from build123d import *

# Parameters (mm, degrees)
SKETCH1_R           = 1.5
SKETCH1_W           = 15.5
SKETCH1_H           = 15.5
BOSS_EXTRUDE1_DEPTH = 1.6
CUT_EXTRUDE2_DEPTH  = 91.713045172
FILLET2_R           = 3
FILLET3_R           = 3


with BuildPart() as part:
    # Sketch1 → Boss-Extrude1 (new body)
    with BuildSketch(Plane.XY):
        with BuildLine():
            Line((80.807032999, -9.202000204), (80.807032999, 37.709242496))
            ThreePointArc((80.807032999, 37.709242496), (79.927673142, 39.831242844), (77.805109389, 40.709241907))
            Line((77.805109389, 40.709241907), (-72.154484411, 40.613083107))
            ThreePointArc((-72.154484411, 40.613083107), (-74.271159988, 39.737121752), (-75.152545414, 37.622699011))
            Line((-75.152545414, 37.622699011), (-75.383320814, -34.379217889))
            ThreePointArc((-75.383320814, -34.379217889), (-74.508053368, -36.506751286), (-72.383336219, -37.388833194))
            Line((-72.383336219, -37.388833194), (-25.613726719, -37.388833194))
            ThreePointArc((-25.613726719, -37.388833194), (-25.488077715, -37.391465627), (-25.362649219, -37.399358309))
            Line((-25.362649219, -37.399358309), (19.631715181, -41.178308109))
            ThreePointArc((19.631715181, -41.178308109), (19.757143676, -41.18620079), (19.88279268, -41.188833223))
            Line((19.88279268, -41.188833223), (68.14475528, -41.188833223))
            ThreePointArc((68.14475528, -41.188833223), (69.898886106, -40.622559803), (70.990805162, -39.137516598))
            Line((70.990805162, -39.137516598), (80.653082862, -10.150683598))
            ThreePointArc((80.653082862, -10.150683598), (80.768295364, -9.682546983), (80.807032999, -9.202000204))
        make_face()
        with Locations((-19.612967014, -21.188833189)):
            Circle(SKETCH1_R, mode=Mode.SUBTRACT)
        with Locations((7.057032986, -25.938833189)):
            Circle(SKETCH1_R, mode=Mode.SUBTRACT)
        with Locations((43.657032986, 35.811166811)):
            Circle(SKETCH1_R, mode=Mode.SUBTRACT)
        with Locations((-70.817967014, -7.888833189)):
            Circle(SKETCH1_R, mode=Mode.SUBTRACT)
        with Locations((57.907032986, -7.888833189)):
            Circle(SKETCH1_R, mode=Mode.SUBTRACT)
        with Locations((-51.342967014, 18.711166811)):
            Circle(SKETCH1_R, mode=Mode.SUBTRACT)
        with Locations((-64.642967014, 30.111166811)):
            Rectangle(SKETCH1_W, SKETCH1_H, mode=Mode.SUBTRACT)
        with Locations((-45.642967014, 30.111166811)):
            Rectangle(SKETCH1_W, SKETCH1_H, mode=Mode.SUBTRACT)
        with Locations((-26.642967014, 30.111166811)):
            Rectangle(SKETCH1_W, SKETCH1_H, mode=Mode.SUBTRACT)
        with Locations((-7.642967014, 30.111166811)):
            Rectangle(SKETCH1_W, SKETCH1_H, mode=Mode.SUBTRACT)
        with Locations((11.357032986, 30.111166811)):
            Rectangle(SKETCH1_W, SKETCH1_H, mode=Mode.SUBTRACT)
        with Locations((30.357032986, 30.111166811)):
            Rectangle(SKETCH1_W, SKETCH1_H, mode=Mode.SUBTRACT)
        with Locations((-62.267967014, 11.111166811)):
            Rectangle(SKETCH1_W, SKETCH1_H, mode=Mode.SUBTRACT)
        with Locations((-40.892967014, 11.111166811)):
            Rectangle(SKETCH1_W, SKETCH1_H, mode=Mode.SUBTRACT)
        with Locations((-21.892967014, 11.111166811)):
            Rectangle(SKETCH1_W, SKETCH1_H, mode=Mode.SUBTRACT)
        with Locations((-2.892967014, 11.111166811)):
            Rectangle(SKETCH1_W, SKETCH1_H, mode=Mode.SUBTRACT)
        with Locations((16.107032986, 11.111166811)):
            Rectangle(SKETCH1_W, SKETCH1_H, mode=Mode.SUBTRACT)
        with Locations((35.107032986, 11.111166811)):
            Rectangle(SKETCH1_W, SKETCH1_H, mode=Mode.SUBTRACT)
        with Locations((-57.517967014, -7.888833189)):
            Rectangle(SKETCH1_W, SKETCH1_H, mode=Mode.SUBTRACT)
        with Locations((-31.392967014, -7.888833189)):
            Rectangle(SKETCH1_W, SKETCH1_H, mode=Mode.SUBTRACT)
        with Locations((-12.392967014, -7.888833189)):
            Rectangle(SKETCH1_W, SKETCH1_H, mode=Mode.SUBTRACT)
        with Locations((6.607032986, -7.888833189)):
            Rectangle(SKETCH1_W, SKETCH1_H, mode=Mode.SUBTRACT)
        with Locations((25.607032986, -7.888833189)):
            Rectangle(SKETCH1_W, SKETCH1_H, mode=Mode.SUBTRACT)
        with Locations((44.607032986, -7.888833189)):
            Rectangle(SKETCH1_W, SKETCH1_H, mode=Mode.SUBTRACT)
        with Locations((-62.267967014, -26.888833189)):
            Rectangle(SKETCH1_W, SKETCH1_H, mode=Mode.SUBTRACT)
        with Locations((-38.612967014, -26.888833189)):
            Rectangle(SKETCH1_W, SKETCH1_H, mode=Mode.SUBTRACT)
        with Locations((26.057032986, -30.688833189)):
            Rectangle(SKETCH1_W, SKETCH1_H, mode=Mode.SUBTRACT)
        with Locations((55.057032986, -30.688833189)):
            Rectangle(SKETCH1_W, SKETCH1_H, mode=Mode.SUBTRACT)
    extrude(amount=BOSS_EXTRUDE1_DEPTH)

    # Sketch3 → Cut-Extrude2 (cut, through all)
    with BuildSketch(Plane.XY.offset(1.6)):
        Polygon((47.443249451, 42.560753869), (47.443249451, 3.300099698), (61.120116682, 3.300099698), (61.120116682, -19.548313794), (65.786341973, -19.548313794), (65.786341973, -41.188833223), (73.358886795, -43.51481274), (105.294000543, 60.45432308), align=None)
    extrude(amount=-CUT_EXTRUDE2_DEPTH, mode=Mode.SUBTRACT)

    # Fillet2
    fillet2_edges = [part.edges().sort_by_distance(p)[0] for p in [
        (47.443249451, 40.689772929, 0.8),
        (65.786341973, -19.548313794, 0.8),
        (61.120116682, 3.300099698, 0.8),
    ]]
    fillet(fillet2_edges, radius=FILLET2_R)

    # Fillet3
    fillet3_edges = [part.edges().sort_by_distance(p)[0] for p in [
        (65.786341973, -41.188833223, 0.8),
    ]]
    fillet(fillet3_edges, radius=FILLET3_R)


solid = part.part
Read the model definition and answer for the solid it produces. Units are mm, in the model's axes. Round coordinates to 2 decimals unless told otherwise and drop trailing zeros. Order: outer loops, then holes, each group sorted by start corner. A loop starts at its lowest first (then second) coordinate and runs counter-clockwise, first axis right, second up.
1) Straight lines are drawn through the part: L1, parallel to Y at x = -59, z = 1.4; L2, parallel to Y at x = -27.5, z = 1.35; L3, parallel to X at y = -31.5, z = 0.6. For each, find the intervals that lie inside material, in ascending order.
2) The mould has two halves that part along X. Classify faces 1 (the face through (-74.25, 39.76, 0.79)), 2 (the face through (-52.533, 17.798, 0.789)), 3 (the face through (-6, -18, 0)): released by +X, released by -X, zero draft, split by the parting line, or undercut.
3) The part is cut by section A-A on y = -12.5. Write down the section's boundary in (x, z), plus the area to 3 significant figures.
4) The part is cut by section B-B on x = 1.5. Write down the section's boundary in (y, z).
5) Flat-ended cylindrical pins translate along their axes: pin 1 (0.8 mm diameter, centred on x = -59.5, z = 0.5, fed in from +Y); pin 2 (0.5 mm diameter, centred on x = 50.5, z = 1, fed in from +Y); pin 3 (0.8 mm diameter, centred on y = 10, z = 1, fed in from -X). Find the tip coordinate at first contact, or state that the pin passes through.
6) The part is cut by section D-D on z = 1.15. Give the number of separate pieces and of enclosed holes in the cut face, plus the area to 3 significant figures.
7) The part is cut by section C-C on y = -3.5. Write down the section's boundary in (x, z).
Resolved:
1. L1: y = -37.39 to -34.64, -19.14 to -15.64, -0.14 to 3.36, 18.86 to 22.36, 37.86 to 40.62
1. L2: y = -37.39 to -15.64, -0.14 to 3.36, 18.86 to 22.36, 37.86 to 40.64
1. L3: x = -75.37 to -70.02, -54.52 to -46.36, -30.86 to 18.31, 33.81 to 47.31, 62.81 to 65.79
2. face 1: released by -X
2. face 2: undercut
2. face 3: zero draft
3. outline: (-75.31, 0) - (-65.27, 0) - (-65.27, 1.6) - (-75.31, 1.6) - close; (-49.77, 0) - (-39.14, 0) - (-39.14, 1.6) - (-49.77, 1.6) - close; (-23.64, 0) - (-20.14, 0) - (-20.14, 1.6) - (-23.64, 1.6) - close; (-4.64, 0) - (-1.14, 0) - (-1.14, 1.6) - (-4.64, 1.6) - close; (14.36, 0) - (17.86, 0) - (17.86, 1.6) - (14.36, 1.6) - close; (33.36, 0) - (36.86, 0) - (36.86, 1.6) - (33.36, 1.6) - close; (52.36, 0) - (61.12, 0) - (61.12, 1.6) - (52.36, 1.6) - close
3. area: 69.5 mm2
4. outline: (-39.66, 0) - (-15.64, 0) - (-15.64, 1.6) - (-39.66, 1.6) - close; (-0.14, 0) - (3.36, 0) - (3.36, 1.6) - (-0.14, 1.6) - close; (18.86, 0) - (40.66, 0) - (40.66, 1.6) - (18.86, 1.6) - close
5. pin 1: stops at y = 40.62
5. pin 2: stops at y = 3.3
5. pin 3: stops at x = -75.24
6. separate pieces: 1
6. enclosed holes: 28
6. area: 5,140 mm2
7. outline: (-75.28, 0) - (-65.27, 0) - (-65.27, 1.6) - (-75.28, 1.6) - close; (-49.77, 0) - (-39.14, 0) - (-39.14, 1.6) - (-49.77, 1.6) - close; (-23.64, 0) - (-20.14, 0) - (-20.14, 1.6) - (-23.64, 1.6) - close; (-4.64, 0) - (-1.14, 0) - (-1.14, 1.6) - (-4.64, 1.6) - close; (14.36, 0) - (17.86, 0) - (17.86, 1.6) - (14.36, 1.6) - close; (33.36, 0) - (36.86, 0) - (36.86, 1.6) - (33.36, 1.6) - close; (52.36, 0) - (61.12, 0) - (61.12, 1.6) - (52.36, 1.6) - close
